The listing builds one solid part. Answer for the finished solid, in the listing's coordinates (mm). Face numbers are marked on the shaded views. Give positions to 0.01 mm unless a question says otherwise; leave off trailing zeros. Write each loop counter-clockwise with the first axis right and the second up, starting at its lowest first coordinate (ties: lowest second). Pieces come first, ordered by that corner, then holes.
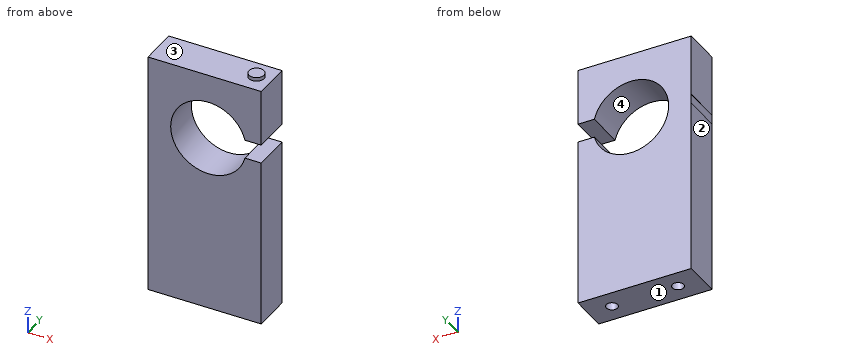
Solid Edge part; units mm, degrees
sketch "Sketch1" plane through (0, 0, 0) normal (0, -1, 0) x (1, 0, 0)
  line L0 (-30, 130) -> (30, 130)
  line L1 (30, 130) -> (30, 100)
  line L2 (30, 100) -> (21.3649, 100)
  line L3 (30, 90) -> (21.3649, 90)
  line L4 (30, 0) -> (30, 90)
  line L5 (-30, 0) -> (30, 0)
  line L6 (-30, 130) -> (-30, 0)
  arc A0 (21.3649, 90) -> (21.3649, 100) centre (2, 95) cw
extrude "Protrusion1" add sketch "Sketch1" along normal mid plane 20
hole "Agujero_1" at (17.5, 0, 0) direction (0, 0, 1) diameter 6 depth 30 tip angle 118
hole "Hole1" at (-17.5, 0, 0) direction (0, 0, 1) diameter 6 depth 30 tip angle 118
sketch "Sketch2" plane through (0, 0, 130) normal (0, 0, 1) x (1, 0, 0)
  circle A0 centre (22, 0) radius 4
extrude "ProtrusiónExtruida_2" add sketch "Sketch2" along normal blind 2
sketch "Sketch3" plane through (-30, 0, 65) normal (-1, 0, 0) x (0, 0, -1)
  line L0 (-32.5, 10) -> (-32.5, -10)
  line L1 (-32.5, -10) -> (-27.5, -10)
  line L2 (-27.5, -10) -> (-27.5, 10)
  line L3 (-27.5, 10) -> (-32.5, 10)
extrude "VaciadoExtruido_1" cut sketch "Sketch3" against normal blind 0.05
Item 1: A cutting plane is placed at C-C, the plane x = 23. Give the vertices of the cut face in (y, z).
Conclusion:
outline: (-10, 0) - (10, 0) - (10, 90) - (-10, 90) - close; (-10, 100) - (10, 100) - (10, 130) - (3.87, 130) - (3.87, 132) - (-3.87, 132) - (-3.87, 130) - (-10, 130) - close
Item 2: Consider probe 1 along X at (y, z) = (0, 20.5); probe 2 along Z at (x, y) = (23, 0.25); probe 3 along Z at (x, y) = (2, 2.5). Determine where each line is inside the solid, lowest interval first.
Conclusion:
probe 1: x = -30 to -20.5, -14.5 to 14.5, 20.5 to 30
probe 2: z = 0 to 90, 100 to 132
probe 3: z = 0 to 75, 115 to 130
Item 3: A cutting plane is placed at A-A, the plane y = -5.5. Give the vertices of the cut face in (x, z), plus the area to 3 significant figures.
Conclusion:
outline: (-30, 0) - (30, 0) - (30, 90) - (21.36, 90) arc R20 cw (long way) to (21.36, 100) - (30, 100) - (30, 130) - (-30, 130) - (-30, 97.5) - (-29.95, 97.5) - (-29.95, 92.5) - (-30, 92.5) - close
area: 6,460 mm2
Item 4: Determine the mould class of the marked faces 1, 2, 3 and 4 for opening direction Z: pulls with the +Z half, pulls with the -Z half, needs draft (parallel to the pull), parting line crosses it, or undercut.
Conclusion:
face 1: pulls with the -Z half
face 2: needs draft
face 3: pulls with the +Z half
face 4: undercut
Item 5: A cutting plane is placed at D-D, the plane z = 27.5. Give the vertices of the cut face in (x, y).
Conclusion:
outline: (-30, -10) - (30, -10) - (30, 10) - (-30, 10) - close; hole circle Ø6 at (-17.5, 0); hole circle Ø6 at (17.5, 0)
Item 6: A cutting plane is placed at B-B, the plane z = 78.5. Give the vertices of the cut face in (x, y), plus the area to 3 significant figures.
Conclusion:
outline: (-30, -10) - (-9.3, -10) - (-9.3, 10) - (-30, 10) - close; (13.3, -10) - (30, -10) - (30, 10) - (13.3, 10) - close
area: 748 mm2
Item 7: This flat-tipped pin is pushed along its axis until it touches: P1, Ø1.5, axis at x = -15, y = 1, coming from the +Z side. Where does it stop, or does it pass through?
Conclusion:
P1: stops at z = 130
